```python
from build123d import *

# Parameters (mm, degrees)
BOSS_EXTRUDE2_DEPTH = 5
BOSS_EXTRUDE3_DEPTH = 40
SKETCH4_R           = 17.5
CUT_EXTRUDE1_DEPTH  = 40
SKETCH5_R           = 26
SKETCH5_R_2         = 23.5
BOSS_EXTRUDE4_DEPTH = 7
SKETCH6_R           = 36
SKETCH6_R_2         = 26
BOSS_EXTRUDE5_DEPTH = 19


with BuildPart() as part:
    # Sketch1 → Boss-Extrude2 (new body)
    with BuildSketch(Plane(origin=(0, 0, 0), x_dir=(1, 0, 0), z_dir=(0, 1, 0))):
        with BuildLine():
            Line((122, -183), (0, -183))
            Line((0, -183), (0, 2))
            ThreePointArc((0, 2), (61, 63), (122, 2))
            Line((122, 2), (122, -183))
        make_face()
    extrude(amount=BOSS_EXTRUDE2_DEPTH)

    # Sketch3 → Boss-Extrude3 (add)
    with BuildSketch(Plane(origin=(0, 5, 0), x_dir=(1, 0, 0), z_dir=(0, 1, 0))):
        with BuildLine():
            Line((122, -183), (122, 2))
            ThreePointArc((122, 2), (61, 63), (0, 2))
            Line((0, 2), (0, -183))
            Line((0, -183), (122, -183))
        make_face()
        with BuildLine():
            Line((5, -178), (5, 2))
            ThreePointArc((5, 2), (61, 58), (117, 2))
            Line((117, 2), (117, -178))
            Line((117, -178), (5, -178))
        make_face(mode=Mode.SUBTRACT)
    extrude(amount=BOSS_EXTRUDE3_DEPTH)

    # Sketch4 → Cut-Extrude1 (cut)
    with BuildSketch(Plane(origin=(0, 5, 0), x_dir=(1, 0, 0), z_dir=(0, 1, 0))):
        with Locations(Location((61, 2, 0), (0, 0, 270))):
            Circle(SKETCH4_R)
    extrude(amount=-CUT_EXTRUDE1_DEPTH, mode=Mode.SUBTRACT)

    # Sketch5 → Boss-Extrude4 (add)
    with BuildSketch(Plane(origin=(0, 5, 0), x_dir=(1, 0, 0), z_dir=(0, 1, 0))):
        with Locations(Location((61, 2, 0), (0, 0, 270))):
            Circle(SKETCH5_R)
        with Locations(Location((61, 2, 0), (0, 0, 270))):
            Circle(SKETCH5_R_2, mode=Mode.SUBTRACT)
    extrude(amount=BOSS_EXTRUDE4_DEPTH)

    # Sketch6 → Boss-Extrude5 (add)
    with BuildSketch(Plane(origin=(0, 5, 0), x_dir=(1, 0, 0), z_dir=(0, 1, 0))):
        with Locations(Location((61, 2, 0), (0, 0, 270))):
            Circle(SKETCH6_R)
        with Locations(Location((61, 2, 0), (0, 0, 270))):
            Circle(SKETCH6_R_2, mode=Mode.SUBTRACT)
    extrude(amount=BOSS_EXTRUDE5_DEPTH)


solid = part.part
```
Here's how the part is built. I have some questions about the finished solid (model axes, mm). A direction names the side the tool comes from. Round coordinates to 2 decimals unless told otherwise and drop trailing zeros. Loops run counter-clockwise (first coordinate to the right, second up) from the corner with the lowest first, then second, coordinate; pieces in that order, holes last.
1. Thinking about a two-plate mould opening in Z: for faces 1 (the face through (38, 12, -8)), 2 (the face through (0, 22, 89)), 3 (the face through (60, 22, 183)), 4 (the face through (96.694, 14.367, -6.686)), which applies, released by +Z, released by -Z, zero draft, split by the parting line, or undercut?
Answers:
face 1: undercut
face 2: zero draft
face 3: released by +Z
face 4: undercut
2. For faces 5 (the face through (61, 5, -20)), 6 (the face through (62.341, 22.185, -62.985)), which set-ups out of +Z, -Z, +X, -X, +Y, -Y let a thin tool reach every point of the face, with its end or its side?
Answers:
face 5: +Y
face 6: -Z, +Y, -Y
3. Suppose I cut it at C-C, the plane x = 61. Please give me the cut outline in (y, z), and give its area (3 significant figures).
Answers:
outline: (0, -63) - (45, -63) - (45, -58) - (5, -58) - (5, -38) - (24, -38) - (24, -28) - (12, -28) - (12, -25.5) - (5, -25.5) - (5, -19.5) - (0, -19.5) - close; (0, 15.5) - (5, 15.5) - (5, 21.5) - (12, 21.5) - (12, 24) - (24, 24) - (24, 34) - (5, 34) - (5, 178) - (45, 178) - (45, 183) - (0, 183) - close
area: 1,870 mm2
4. If I drill on probe 1 along X at (y, z) = (10.75, -2); probe 2 along X at (y, z) = (18, -2); probe 3 along X at (y, z) = (5.5, 172), over which ranges is the centre line in solid material (lowest first)?
Answers:
probe 1: x = 0 to 5, 25 to 37.5, 84.5 to 97, 117 to 122
probe 2: x = 0 to 5, 25 to 35, 87 to 97, 117 to 122
probe 3: x = 0 to 5, 117 to 122
5. Suppose I cut it at D-D, the plane z = 106.5. Please give me the cut outline in (x, y).
Answers:
outline: (0, 0) - (122, 0) - (122, 45) - (117, 45) - (117, 5) - (5, 5) - (5, 45) - (0, 45) - close
6. Will these pins go through, and if not, where does the flat tip stop? pin 1 (10 mm diameter, centred on x = 44, y = 37.5, fed in from -Z); pin 2 (12 mm diameter, centred on x = 59.5, z = 142.5, fed in from +Y); pin 3 (4 mm diameter, centred on x = 36.5, y = 32.5, fed in from -Z).
Answers:
pin 1: stops at z = -61.81
pin 2: stops at y = 5
pin 3: stops at z = -58.7
7. Suppose I cut it at B-B, the plane y = 35. Please give me the cut outline in (x, z), and give its area (3 significant figures).
Answers:
outline: (0, -2) arc R61 ccw to (122, -2) - (122, 183) - (0, 183) - close; hole (5, -2) arc R56 ccw to (117, -2) - (117, 178) - (5, 178) - close
area: 3,330 mm2
8. Suppose I cut it at A-A, the plane y = 18. Please give me the cut outline in (x, z).
Answers:
outline: (0, -2) arc R61 ccw to (122, -2) - (122, 183) - (0, 183) - close; circle Ø72 at (61, -2); hole (5, -2) arc R56 ccw to (117, -2) - (117, 178) - (5, 178) - close; hole circle Ø52 at (61, -2)
